Here's the drawing with two shaded views (mm, measured from the low corner). I have some questions. A direction names the side the tool comes from. Round coordinates to 2 decimals unless told otherwise and drop trailing zeros. Loops run counter-clockwise (first coordinate to the right, second up) from the corner with the lowest first, then second, coordinate; pieces in that order, holes last. Notation, with made-up numbers: M 28,89 L 65,89 A20 ccw 65,96 Z; hole C 36,51 d7. An arc over 180 degrees is marked long. Answer as CSV lines item,"result".
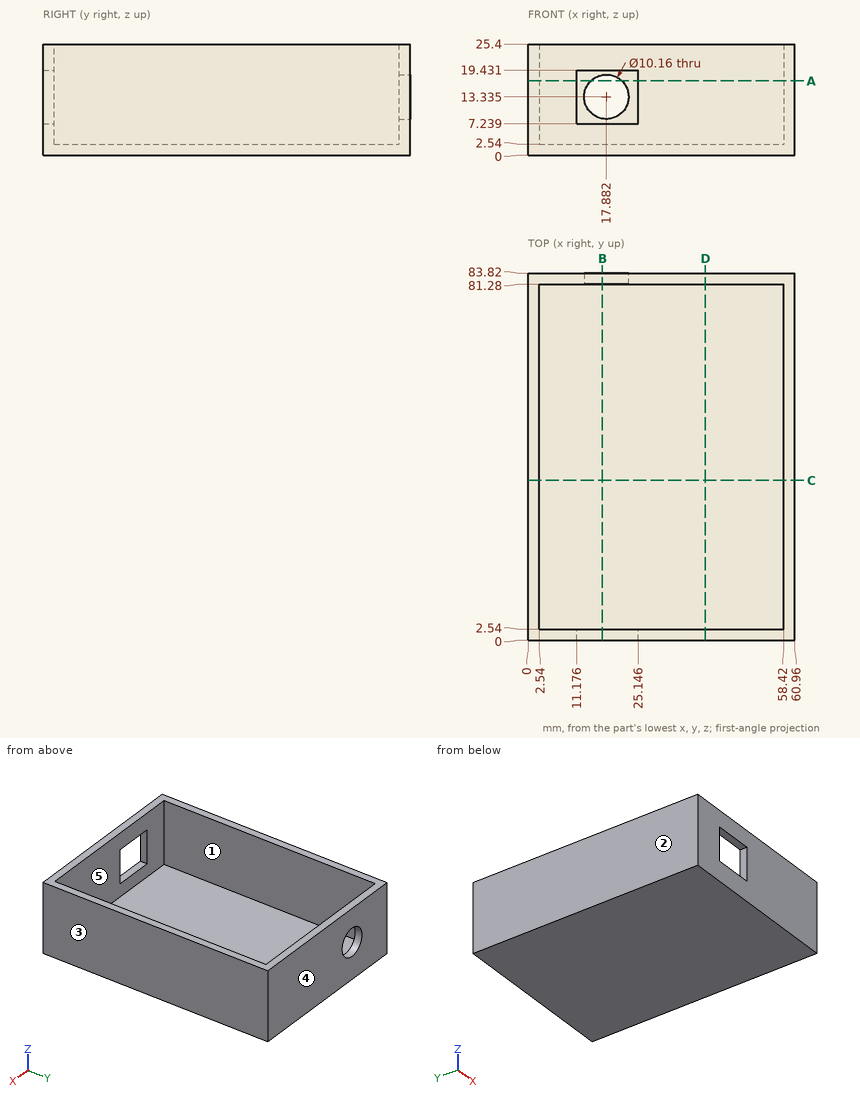
1. For P1, Ø8, axis at x = 50.5, y = 37.5, coming from the +Z side; P2, Ø1, axis at y = 66, z = 6, coming from the -X side; P3, Ø8, axis at x = 17.88, z = 13.34, coming from the +Y side, each with a flat end and sliding along its axis, tell me the tip position at first contact or that it passes through.
Evaluation:
P1,"stops at z = 2.54"
P2,"stops at x = 0"
P3,"passes through"
2. If I drill on line 1 (X direction, y = 34.5, z = 3); line 2 (Y direction, x = 31.5, z = 17.75); line 3 (Z direction, x = 25, y = 67), over which ranges is the centre line in solid material (lowest first)? Write a range as [from, to].
Evaluation:
line 1,"x = [0, 2.54], [58.42, 60.96]"
line 2,"y = [0, 2.54], [81.28, 83.82]"
line 3,"z = [0, 2.54]"
3. I want a section at A-A, the plane z = 17. Please give me the cut outline in (x, y).
Evaluation:
outline,"M 0,0 L 11.18,0 L 11.18,2.54 L 2.54,2.54 L 2.54,81.28 L 14.36,81.28 L 14.36,83.82 L 0,83.82 Z; M 21.4,81.28 L 58.42,81.28 L 58.42,2.54 L 25.15,2.54 L 25.15,0 L 60.96,0 L 60.96,83.82 L 21.4,83.82 Z"
4. Which directions (+Z, -Z, +X, -X, +Y, -Y) give clear straight access to the entire face, cutting with the end or side of a thin tool? Please do the marked faces 1 and 2.
Evaluation:
face 1,"+Z"
face 2,"+Z, -Z, -X, +Y, -Y"
5. We'd pull the mould along X, two halves only. Please class the marked faces 3, 4 and 5: pulls with the +X half, pulls with the -X half, needs draft (parallel to the pull), parting line crosses it, or undercut.
Evaluation:
face 3,"pulls with the +X half"
face 4,"needs draft"
face 5,"undercut"
6. I want a section at C-C, the plane y = 36.5. Please give me the cut outline in (x, z).
Evaluation:
outline,"M 0,0 L 60.96,0 L 60.96,25.4 L 58.42,25.4 L 58.42,2.54 L 2.54,2.54 L 2.54,25.4 L 0,25.4 Z"
7. I want a section at D-D, the plane x = 40.5. Please give me the cut outline in (y, z), and give its area (3 significant figures).
Evaluation:
outline,"M 0,0 L 83.82,0 L 83.82,25.4 L 81.28,25.4 L 81.28,2.54 L 2.54,2.54 L 2.54,25.4 L 0,25.4 Z"
area,"329 mm²"
8. I want a section at B-B, the plane x = 17. Please give me the cut outline in (y, z).
Evaluation:
outline,"M 0,0 L 83.82,0 L 83.82,8.33 L 81.28,8.33 L 81.28,2.54 L 2.54,2.54 L 2.54,7.24 L 0,7.24 Z; M 0,19.43 L 2.54,19.43 L 2.54,25.4 L 0,25.4 Z; M 81.28,18.34 L 83.82,18.34 L 83.82,25.4 L 81.28,25.4 Z"
